```python
from build123d import *

# Parameters (mm, degrees)
SKETCH_1_R          = 2
SKETCH_1_W          = 3
SKETCH_1_H          = 8
SKETCH_1_W_2        = 8
SKETCH_1_H_2        = 3
EXTRUDE_1_DEPTH     = 3
SKETCH_2_W          = 60
SKETCH_2_H          = 50
CUT_EXTRUDE_1_DEPTH = 10
SKETCH_3_R          = 11
CUT_EXTRUDE_2_DEPTH = 10


with BuildPart() as part:
    # 草图1 → 凸台-拉伸1 (new body)
    with BuildSketch(Plane(origin=(0, 0, 0), x_dir=(1, 0, 0), z_dir=(0, 1, 0))):
        Polygon((-30, -27.5), (-10, -72.5), (10, -72.5), (30, -27.5), (30, 27.5), (-30, 27.5), align=None)
        with Locations(Location((0, -37.5, 0), (0, 0, 270))):
            Circle(SKETCH_1_R, mode=Mode.SUBTRACT)
        with Locations(Location((0, -57.5, 0), (0, 0, 270))):
            Circle(SKETCH_1_R, mode=Mode.SUBTRACT)
        with Locations((-24, 13.5)):
            Rectangle(SKETCH_1_W, SKETCH_1_H, mode=Mode.SUBTRACT)
        with Locations((-24, -13.5)):
            Rectangle(SKETCH_1_W, SKETCH_1_H, mode=Mode.SUBTRACT)
        with Locations((13.5, 24)):
            Rectangle(SKETCH_1_W_2, SKETCH_1_H_2, mode=Mode.SUBTRACT)
        with Locations((-13.5, 24)):
            Rectangle(SKETCH_1_W_2, SKETCH_1_H_2, mode=Mode.SUBTRACT)
        with Locations((-13.5, -24)):
            Rectangle(SKETCH_1_W_2, SKETCH_1_H_2, mode=Mode.SUBTRACT)
        with Locations((13.5, -24)):
            Rectangle(SKETCH_1_W_2, SKETCH_1_H_2, mode=Mode.SUBTRACT)
        with Locations((24, 13.5)):
            Rectangle(SKETCH_1_W, SKETCH_1_H, mode=Mode.SUBTRACT)
        with Locations((24, -13.5)):
            Rectangle(SKETCH_1_W, SKETCH_1_H, mode=Mode.SUBTRACT)
    extrude(amount=EXTRUDE_1_DEPTH)

    # 草图2 → 切除-拉伸1 (cut)
    with BuildSketch(Plane(origin=(0, 3, 0), x_dir=(1, 0, 0), z_dir=(0, 1, 0))):
        with Locations((0, -52.5)):
            Rectangle(SKETCH_2_W, SKETCH_2_H)
    extrude(amount=-CUT_EXTRUDE_1_DEPTH, mode=Mode.SUBTRACT)

    # 草图3 → 切除-拉伸2 (cut)
    with BuildSketch(Plane(origin=(0, 3, 0), x_dir=(1, 0, 0), z_dir=(0, 1, 0))):
        with Locations(Location((0, 0, 0), (0, 0, 270))):
            Circle(SKETCH_3_R)
    extrude(amount=-CUT_EXTRUDE_2_DEPTH, mode=Mode.SUBTRACT)


solid = part.part
```
Input: part model. Units: mm. Frame: model coordinates. A direction names the side the tool comes from. Round coordinates to 2 decimals unless told otherwise and drop trailing zeros. Loops run counter-clockwise (first coordinate to the right, second up) from the corner with the lowest first, then second, coordinate; pieces in that order, holes last. Notation, with made-up numbers: (27, 69) - (44, 69) arc R30 cw to (44, 101) - close; hole circle Ø3 at (70.25, 50). An arc over 180 degrees is marked (long way). One line per item, written item: value. Start each with the question number.
(1) Contact query for a flat-ended pin moving along its axis: P1, Ø3, axis at x = 21, z = 6.5, coming from the -Y side. Output: stop coordinate, or through.
(2) Section B-B, the plane x = 0. Return loops of the section in (y, z).
(3) Draft query along X for faces 3 (the flat face through (0, 1, -27.5)), 4 (the flat face through (-30, 1, 0)), 5 (the flat face through (-14, 1, 25.5)). Return one class per face: +X half, -X half, draft (parallel to the pull), parting line (faces both ways), or undercut.
(4) Section A-A, the plane z = 0. Return loops of the section in (x, y), plus the area to 3 significant figures.
(5) Section C-C, the plane z = 23.5. Return loops of the section in (x, y), plus the area to 3 significant figures.
(6) Ray query, line 1 (Z direction, x = 15.5, y = 1.65); line 2 (X direction, y = 1.3, z = 0); line 3 (X direction, y = 1, z = -3). Return the intervals inside material, ascending. Write a range as [from, to].
(7) Access query for faces 1 (the flat face through (24, 1, -17.5)), 2 (the flat face through (30, 1, 0)). Directions: +Z, -Z, +X, -X, +Y, -Y. A direction counts if a zero-diameter tool reaches every point of the face in a straight line with its end or side. Return the directions, or none.
(8) Section D-D, the plane z = -14. Return loops of the section in (x, y), plus the area to 3 significant figures.
Results below:
1. P1: y = 0
2. outline: (0, -27.5) - (3, -27.5) - (3, -11) - (0, -11) - close; (0, 11) - (3, 11) - (3, 27.5) - (0, 27.5) - close
3. face 3: draft
3. face 4: -X half
3. face 5: undercut
4. outline: (-30, 0) - (-11, 0) - (-11, 3) - (-30, 3) - close; (11, 0) - (30, 0) - (30, 3) - (11, 3) - close
4. area: 114 mm^2
5. outline: (-30, 0) - (-17.5, 0) - (-17.5, 3) - (-30, 3) - close; (-9.5, 0) - (9.5, 0) - (9.5, 3) - (-9.5, 3) - close; (17.5, 0) - (30, 0) - (30, 3) - (17.5, 3) - close
5. area: 132 mm^2
6. line 1: [-27.5, -25.5], [-22.5, 22.5], [25.5, 27.5]
6. line 2: [-30, -11], [11, 30]
6. line 3: [-30, -10.58], [10.58, 30]
7. face 1: +Y, -Y
7. face 2: +Z, -Z, +X, +Y, -Y
8. outline: (-30, 0) - (-25.5, 0) - (-25.5, 3) - (-30, 3) - close; (-22.5, 0) - (22.5, 0) - (22.5, 3) - (-22.5, 3) - close; (25.5, 0) - (30, 0) - (30, 3) - (25.5, 3) - close
8. area: 162 mm^2
